Geometry: final body of the model. Coordinates: model frame, mm. A direction names the side the tool comes from. Coordinates: 2 decimals unless noted, no trailing zeros. Loops run counter-clockwise (first coordinate to the right, second up) from the corner with the lowest first, then second, coordinate; pieces in that order, holes last. Notation, with made-up numbers: (58.25, 38) - (113.25, 38) arc R17 ccw to (113.25, 48) - close; hole circle Ø11 at (-28.5, 39). An arc over 180 degrees is marked (long way). Answer in a Markdown table with one row per item.
Autodesk Inventor part; units mm, degrees
ref_plane "YZ Plane" through (0, 0, 0) normal (1, 0, 0) x (0, 1, 0)
ref_plane "XZ Plane" through (0, 0, 0) normal (0, 1, 0) x (-1, 0, 0)
ref_plane "XY Plane" through (0, 0, 0) normal (0, 0, 1) x (1, 0, 0)
sketch "Szkic1" plane through (0, 0, 0) normal (0, 1, 0) x (-1, 0, 0)
  line L0 (-16.5, 8.5) -> (16.5, 8.5)
  line L1 (16.5, 8.5) -> (16.5, -8.5)
  line L2 (16.5, -8.5) -> (-16.5, -8.5)
  line L3 (-16.5, -8.5) -> (-16.5, 8.5)
  line L4 (-16.5, 8.5) -> (16.5, -8.5) construction
  line L5 (16.5, 8.5) -> (-16.5, -8.5) construction
  line L6 (-17.5, 9.5) -> (17.5, 9.5)
  line L7 (17.5, 9.5) -> (17.5, -9.5)
  line L8 (17.5, -9.5) -> (-17.5, -9.5)
  line L9 (-17.5, -9.5) -> (-17.5, 9.5)
  line L10 (-17.5, 9.5) -> (17.5, -9.5) construction
  line L11 (17.5, 9.5) -> (-17.5, -9.5) construction
  circle A0 centre (0, 0) radius 1.75
  circle A1 centre (0, 0) radius 3.5
  dimension "d0" = 33
  dimension "d1" = 17
  dimension "d2" = 35
  dimension "d3" = 19
  dimension "d4" = 3.5
  dimension "d5" = 7
extrude "Wyciągnięcie proste1" add sketch "Szkic1" along normal blind 6 contours L6 L7 L8 L9
extrude "Wyciągnięcie proste2" add sketch "Szkic1" against normal blind 2 contours L0 L1 L2 L3 | L6 L7 L8 L9 | A1
extrude "Wyciągnięcie proste3" cut sketch "Szkic1" against normal blind 1.8 contours A1
sketch "Szkic2" plane through (17.5, 6, 9.5) normal (1, 0, 0) x (0, 0, -1)
  line L0 (1, -6) -> (1, 0)
  line L1 (18, -6) -> (1, -6)
  line L2 (1, -6) -> (18, -6)
  line L3 (9.5, -6) -> (9.5, 0)
  line L4 (0, 0) -> (19, 0)
  line L5 (9.5, -6) -> (9.5, -3)
  circle A0 centre (9.5, -4.5) radius 2.5
  point P0 (11.5, -6)
  point P1 (7.5, -6)
  dimension "d14" = 5
extrude "Wyciągnięcie proste4" cut sketch "Szkic2" against normal blind 39.25 contours A0 L3 L1 | L3 A0 L1
properties part number "Battery_box"
(1) Cut plane C-C on y = 1. Output: boundary loops of the cut face in (x, z), then the cut area to 3 significant figures.
Verdict:
| item | result |
|---|---|
| outline | (-17.5, -9.5) - (17.5, -9.5) - (17.5, -2.45) - (16.5, -2.45) - (16.5, -8.5) - (-16.5, -8.5) - (-16.5, -2.45) - (-17.5, -2.45) - close; (-17.5, 2.45) - (-16.5, 2.45) - (-16.5, 8.5) - (16.5, 8.5) - (16.5, 2.45) - (17.5, 2.45) - (17.5, 9.5) - (-17.5, 9.5) - close |
| area | 94.2 mm² |
(2) Cut plane D-D on z = 4.25. Output: boundary loops of the cut face in (x, y).
Verdict:
| item | result |
|---|---|
| outline | (-17.5, -2) - (17.5, -2) - (17.5, 6) - (16.5, 6) - (16.5, 0) - (-16.5, 0) - (-16.5, 6) - (-17.5, 6) - close |
(3) Cut plane A-A on x = 0. Output: boundary loops of the cut face in (y, z), then the cut area to 3 significant figures.
Verdict:
| item | result |
|---|---|
| outline | (-2, -9.5) - (6, -9.5) - (6, -8.5) - (0, -8.5) - (0, -3.5) - (-1.8, -3.5) - (-1.8, -1.75) - (-2, -1.75) - close; (-2, 1.75) - (-1.8, 1.75) - (-1.8, 3.5) - (0, 3.5) - (0, 8.5) - (6, 8.5) - (6, 9.5) - (-2, 9.5) - close |
| area | 36.7 mm² |
(4) Access query for faces 4 (the face through (-16.5, 4.3, 0.1)), 5 (the face through (0, -2, 2)). Directions: +Z, -Z, +X, -X, +Y, -Y. A direction counts if a zero-diameter tool reaches every point of the face in a straight line with its end or side. Return the directions, or none.
Verdict:
| item | result |
|---|---|
| face 4 | +Y |
| face 5 | +Z, -Z, +X, -X, -Y |
(5) Ray query, probe 1 along Z at (x, y) = (0, -0.4); probe 2 along Z at (x, y) = (-4.5, 4); probe 3 along X at (y, z) = (4, 6.5). Return the intervals inside material, ascending.
Verdict:
| item | result |
|---|---|
| probe 1 | z = -9.5 to -3.5, 3.5 to 9.5 |
| probe 2 | z = -9.5 to -8.5, 8.5 to 9.5 |
| probe 3 | x = -17.5 to -16.5, 16.5 to 17.5 |
(6) First-contact query: pin 1 Ø5 at (x, z) = (-3.5, -1.5) entering from +Y; pin 2 Ø3 at (x, z) = (0, 0) entering from -Y. Flat tips, straight axial feed; report the tip coordinate or a pass-through.
Verdict:
| item | result |
|---|---|
| pin 1 | stops at y = 0 |
| pin 2 | passes through |
(7) Pull-direction query (Z, two-part tool) for faces 1 (the face through (2, -1.8, -1)), 2 (the face through (-17.5, 5, 0)), 3 (the face through (0, 2, 9.5)); classes: pulls with the +Z half, pulls with the -Z half, needs draft (parallel to the pull), parting line crosses it, or undercut.
Verdict:
| item | result |
|---|---|
| face 1 | undercut |
| face 2 | needs draft |
| face 3 | pulls with the +Z half |
(8) Cut plane B-B on z = 0. Output: boundary loops of the cut face in (x, y), then the cut area to 3 significant figures.
Verdict:
| item | result |
|---|---|
| outline | (-17.5, -2) - (-1.75, -2) - (-1.75, -1.8) - (-3.5, -1.8) - (-3.5, 0) - (-17.5, 0) - close; (-17.5, 4) - (-16.5, 4) - (-16.5, 6) - (-17.5, 6) - close; (1.75, -2) - (17.5, -2) - (17.5, 0) - (3.5, 0) - (3.5, -1.8) - (1.75, -1.8) - close; (16.5, 4) - (17.5, 4) - (17.5, 6) - (16.5, 6) - close |
| area | 60.7 mm² |
